from build123d import *

# Parameters (mm, degrees)
F0_W     = 123
F0_H     = 59
F1_DEPTH = 10
F2_R     = 5
F3_R     = 5
F4_R     = 2.7669489105
F4_R_2   = 2.5059208377
F5_DEPTH = 1
F6_W     = 7.6256990433
F6_H     = 3.5195555538
F7_DEPTH = 0.5
F8_R     = 4.6382964955
F9_DEPTH = 0.5
F10_SIZE = 0.49999


# Not quite as in the source:
# - a fillet or chamfer is up to 0.001 mm smaller than in the source, because OpenCascade refuses the exact size


with BuildPart() as f1:
    # F0 (on Top) → F1 (new body)
    with BuildSketch(Plane.XY):
        Rectangle(F0_W, F0_H)
    extrude(amount=F1_DEPTH)

    # F2
    f2_edges = [f1.edges().sort_by_distance(p)[0] for p in [
        (-61.5, 29.5, 5),
        (61.5, 29.5, 5),
    ]]
    fillet(f2_edges, radius=F2_R)

    # F3
    f3_edges = [f1.edges().sort_by_distance(p)[0] for p in [
        (-61.5, -29.5, 5),
        (61.5, -29.5, 5),
    ]]
    fillet(f3_edges, radius=F3_R)

    # F4 (on face) → F5 (join)
    with BuildSketch(Plane.XZ.offset(29.5)):
        with Locations((37.291161716, 5.468532443)):
            Circle(F4_R)
        with Locations((47.2632274032, 5.468532443)):
            Circle(F4_R_2)
    extrude(amount=F5_DEPTH)

    # F6 (on face) → F7 (join)
    with BuildSketch(Plane.YZ.offset(61.5)):
        with Locations((18.0802661926, 4.9434783868)):
            Rectangle(F6_W, F6_H)
    extrude(amount=F7_DEPTH)

    # F8 (on face) → F9 (cut)
    with BuildSketch(Plane.XY.offset(10)):
        with Locations((-54.5105189085, 0)):
            Circle(F8_R)
    extrude(amount=-F9_DEPTH, mode=Mode.SUBTRACT)

    # F10 (size 0.5 in the source; OpenCascade refuses exactly that, so slightly less here)
    f10_edges = [f1.edges().sort_by_distance(p)[0] for p in [
        (61.5, 0, 10),
        (60.035534, -28.035534, 10),
        (60.035534, 28.035534, 10),
        (0, -29.5, 10),
        (0, 29.5, 10),
        (-60.035534, -28.035534, 10),
        (-60.035534, 28.035534, 10),
        (-61.5, 0, 10),
        (-59.148815, 0, 10),
    ]]
    chamfer(f10_edges, length=F10_SIZE)


solid = f1.part
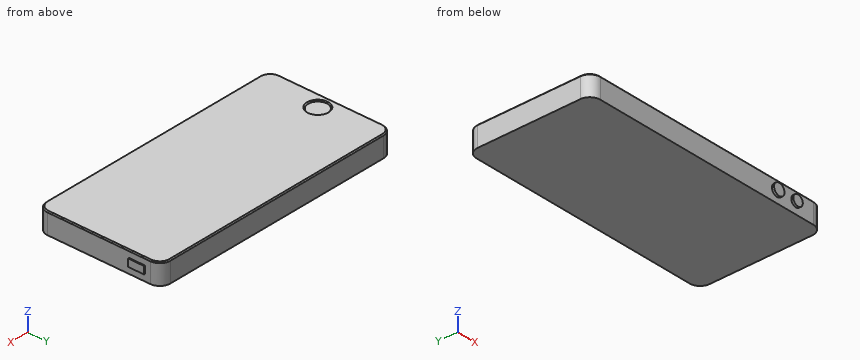
Verification items for the finished model (mm, model axes). Coordinates: 2 decimals unless noted, no trailing zeros. Loops run counter-clockwise (first coordinate to the right, second up) from the corner with the lowest first, then second, coordinate; pieces in that order, holes last. Notation, with made-up numbers: (29, 7.25) -> (88, 7.25) arc R28 ccw to (88, 44.25) -> close; hole circle Ø9 at (30.5, 83). An arc over 180 degrees is marked (long way). Answer as a JSON object with one key per item and string values. Group by question number.
Item 1: Scan lines: probe 1 along Y at (x, z) = (34, 1); probe 2 along X at (y, z) = (-24, 9.25); probe 3 along X at (y, z) = (0, 9.55). Record each from-to range of solid material in increasing order.
Item 2: Sectioned sample at A-A on x = 52. Record the boundary of the cut face in (y, z), plus the area to 3 significant figures.
Item 3: Depth check by flat-ended pin: pin 1 (5 mm diameter, centred on x = 2.5, z = 2, fed in from -Y); pin 2 (4.5 mm diameter, centred on x = -56.5, y = -1, fed in from +Z); pin 3 (2 mm diameter, centred on y = -5, z = 6.5, fed in from +X). Enter the tip coordinate at first touch or a pass-through.
Evaluation:
{
 "1": {"probe 1": "y = -29.5 to 29.5", "probe 2": "x = -61.5 to 61.5", "probe 3": "x = -61.45 to -59.2, -49.82 to 61.45"},
 "2": {"outline": "(-29.5, 0) -> (29.5, 0) -> (29.5, 9.5) -> (29, 10) -> (-29, 10) -> (-29.5, 9.5) -> close", "area": "590 mm²"},
 "3": {"pin 1": "stops at y = -29.5", "pin 2": "stops at z = 9.5", "pin 3": "stops at x = 61.5"}
}
